For this review, use the dimensioned drawing (mm, ordinates from the lowest corner) and the shaded views. Coordinates: 2 decimals unless noted, no trailing zeros. Order: outer loops, then holes, each group sorted by start corner. A loop starts at its lowest first (then second) coordinate and runs counter-clockwise, first axis right, second up. Notation, with made-up numbers: M 1.5,-29 L 19.5,-29 A5 cw 19.5,-21 Z; hole C -33.75,37.25 d1. An arc over 180 degrees is marked long. Answer as CSV lines item,"result". Start each with the question number.
Q1. For P1, Ø1.5, axis at x = 1, y = 3, coming from the -Z side; P2, Ø2, axis at y = 4, z = 4, coming from the +X side; P3, Ø1, axis at y = 0.5, z = 3, coming from the +X side, all flat-tipped, find the tip position at first contact; note any pin that passes through.
Q2. Wall thickness on L1, parallel to Y at x = 2.15, z = 3.75; L2, parallel to X at y = 1.8, z = 10; L3, parallel to X at y = 0.6, z = 5: over which ranges is each line inside the solid? List them lowest first. Write a range as [from, to].
Q3. Consider section A-A on z = 15.25. Write out the cut boundary in (x, y), and give its area (3 significant figures).
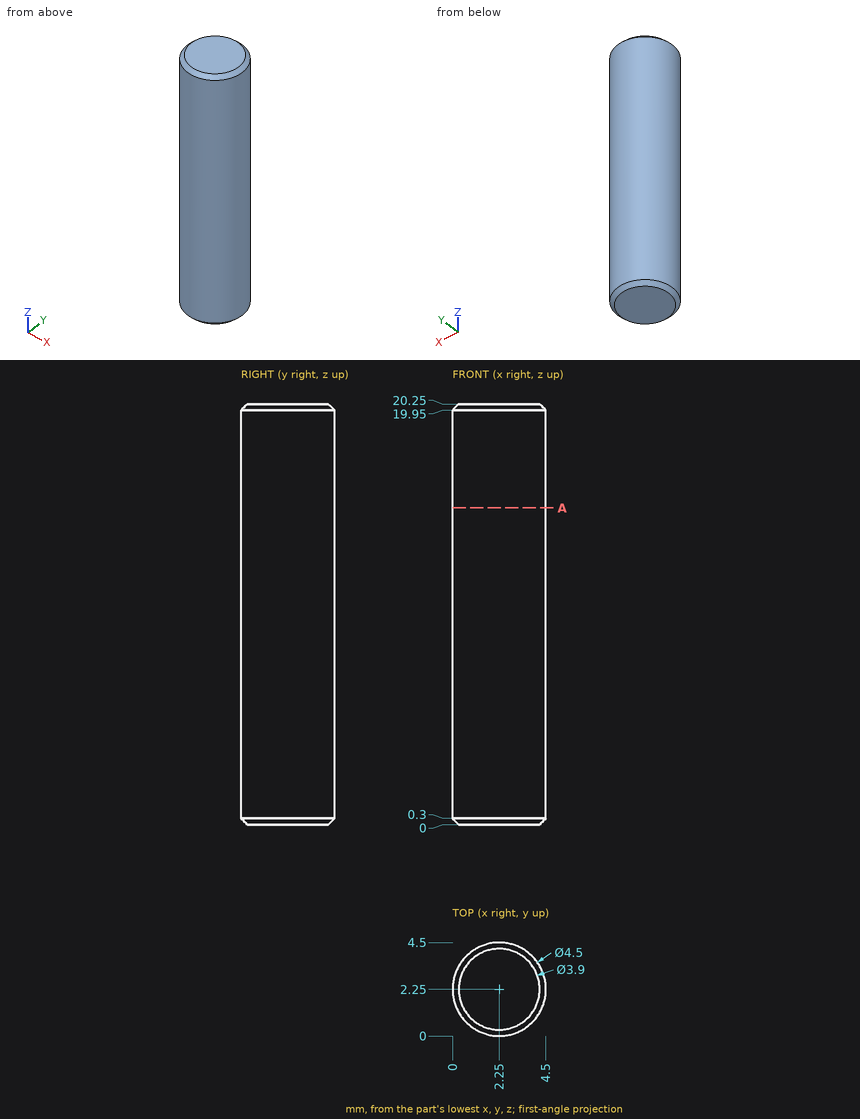
Evaluation:
1,P1,"stops at z = 0"
1,P2,"stops at x = 4.37"
1,P3,"stops at x = 4.12"
2,L1,"y = [0, 4.5]"
2,L2,"x = [0.05, 4.45]"
2,L3,"x = [0.72, 3.78]"
3,outline,"C 2.25,2.25 d4.5"
3,area,"15.9 mm²"
